Source: CAD feature listing. Evaluate the final solid. Frame: model axes, mm. Face numbers are marked on the shaded views. Give positions to 0.01 mm unless a question says otherwise; leave off trailing zeros. Order: outer loops, then holes, each group sorted by start corner. A loop starts at its lowest first (then second) coordinate and runs counter-clockwise, first axis right, second up. Notation, with made-up numbers: M 88.5,37 L 126.5,37 A23 cw 126.5,45 Z; hole C 19.5,23 d7. An arc over 180 degrees is marked long. Use CSV: the item, a comma, the result in double quotes. Start each with the question number.
1. Mould query, pull axis X, two halves, no side actions, for the marked faces 1, 2, 3 and 4. Classes: released by +X, released by -X, zero draft, split by the parting line, or undercut.
2. Section query D-D, the plane x = 6. Return the cut outline in (y, z) (3 decimals).
3. Section query B-B, the plane y = -2. Return the cut outline in (x, z) (3 decimals).
4. Section query C-C, the plane x = 21. Return the cut outline in (y, z) (3 decimals).
5. Section query A-A, the plane z = -63.5. Return the cut outline in (x, y).
6. Pin query (flat end, axial travel): P1, Ø4, axis at x = 27, y = -13, coming from the +Z side; P2, Ø3, axis at x = 50.5, y = -5.5, coming from the +Z side; P3, Ø5, axis at x = 3, y = -13, coming from the +Z side. Return the tip coordinate at first contact, or that it passes through.
7. Line query: line 1 along Z through (x, y) = (-0.5, -1.5) (3 decimals); line 2 along X through (y, z) = (-4.25, -68.5); line 3 along Z through (x, y) = (36, -10.25) (3 decimals). Output: solid intervals per line, ascending. Write a range as [from, to].
from build123d import *

# Parameters (mm, degrees)
F1_DEPTH    = 19.05
F2_T1_DEPTH = 50.8
F2_T3_DEPTH = 36.6217233344


# Not quite as in the source:
# - a fillet or chamfer that OpenCascade refuses, or shapes differently, is made with other operations: its cross-section is extruded or revolved along the edge and cut away or added


with BuildPart() as f1:
    # F0 (on Front) → F1 (new body)
    with BuildSketch(Plane.XZ):
        with BuildLine():
            ThreePointArc((64.3887874714, -38.322173059), (0, -74.93), (-64.3887874714, -38.322173059))
            Line((-64.3887874714, -38.322173059), (-73.66, -38.322173059))
            Line((-73.66, -38.322173059), (-73.66, -135.255))
            Line((-73.66, -135.255), (73.66, -135.255))
            Line((73.66, -135.255), (73.66, -38.322173059))
            Line((73.66, -38.322173059), (64.3887874714, -38.322173059))
        make_face()
    extrude(amount=F1_DEPTH)

    # F2: fillet of radius 6.35 on 6 edges, made by hand

    # F2_s2 → F2_t1 (cut)
    with BuildSketch(Plane.XZ.offset(-15.875)):
        with BuildLine():
            ThreePointArc((67.31, -38.322173059), (71.8001280605, -40.1820449985), (73.66, -44.672173059))
            Line((73.66, -44.672173059), (73.66, -38.322173059))
            Line((73.66, -38.322173059), (67.31, -38.322173059))
        make_face()
        with BuildLine():
            ThreePointArc((-67.31, -38.322173059), (-71.8001280605, -40.1820449985), (-73.66, -44.672173059))
            Line((-73.66, -44.672173059), (-73.66, -38.322173059))
            Line((-73.66, -38.322173059), (-67.31, -38.322173059))
        make_face()
        with BuildLine():
            ThreePointArc((67.31, -135.255), (71.8001280605, -133.3951280605), (73.66, -128.905))
            Line((73.66, -128.905), (73.66, -135.255))
            Line((73.66, -135.255), (67.31, -135.255))
        make_face()
        with BuildLine():
            ThreePointArc((-73.66, -128.905), (-71.8001280605, -133.3951280605), (-67.31, -135.255))
            Line((-67.31, -135.255), (-73.66, -135.255))
            Line((-73.66, -135.255), (-73.66, -128.905))
        make_face()
    extrude(amount=F2_T1_DEPTH, mode=Mode.SUBTRACT)

    # F2_s4 → F2_t3 (cut)
    with BuildSketch(Plane.XZ.offset(-8.7858616672)):
        with BuildLine():
            ThreePointArc((-62.59819994, -41.1821595388), (-64.889752462, -39.0827148628), (-67.9031321383, -38.322173059))
            Line((-67.9031321383, -38.322173059), (-64.3887874714, -38.322173059))
            ThreePointArc((-64.3887874714, -38.322173059), (-63.5095947367, -39.7622468729), (-62.59819994, -41.1821595388))
        make_face()
        with BuildLine():
            ThreePointArc((67.9031321383, -38.322173059), (64.889752462, -39.0827148628), (62.59819994, -41.1821595388))
            ThreePointArc((62.59819994, -41.1821595388), (63.5095947367, -39.7622468729), (64.3887874714, -38.322173059))
            Line((64.3887874714, -38.322173059), (67.9031321383, -38.322173059))
        make_face()
    extrude(amount=F2_T3_DEPTH, mode=Mode.SUBTRACT)


solid = f1.part
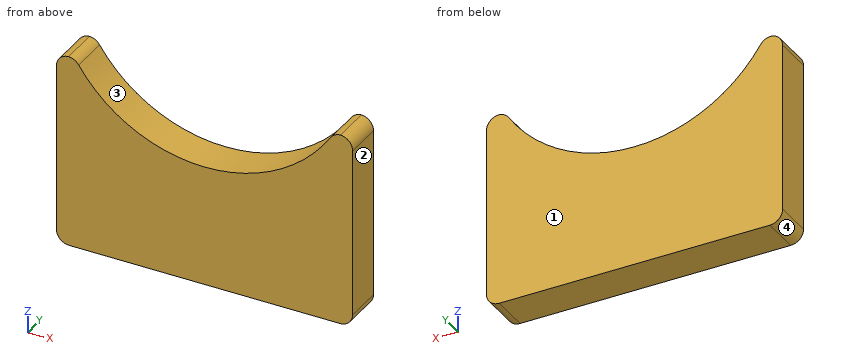
Result set:
1,face 1,"zero draft"
1,face 2,"released by +X"
1,face 3,"undercut"
1,face 4,"released by -X"
2,outline,"M -19.05,-135.255 L 0,-135.255 L 0,-74.689 L -19.05,-74.689 Z"
3,outline,"M -73.66,-128.905 A6.35 ccw -67.31,-135.255 L 67.31,-135.255 A6.35 ccw 73.66,-128.905 L 73.66,-44.672 A6.35 ccw 67.607,-38.329 A6.35 ccw 62.598,-41.182 A74.93 cw -62.598,-41.182 A6.35 ccw -67.607,-38.329 A6.35 ccw -73.66,-44.672 Z"
4,outline,"M -19.05,-135.255 L 0,-135.255 L 0,-71.927 L -19.05,-71.927 Z"
5,outline,"M -73.66,-19.05 L -39.78,-19.05 L -39.78,0 L -73.66,0 Z; M 39.78,-19.05 L 73.66,-19.05 L 73.66,0 L 39.78,0 Z"
6,P1,"z = -69.09"
6,P2,"z = -53.95"
6,P3,"z = -74.73"
7,line 1,"[-135.255, -74.928]"
7,line 2,"[-73.66, -30.37], [30.37, 73.66]"
7,line 3,"[-135.255, -65.715]"
